Here's how the part is built. I have some questions about the finished solid (model axes, mm). A direction names the side the tool comes from. Give positions to 0.01 mm unless a question says otherwise; leave off trailing zeros. Loops run counter-clockwise (first coordinate to the right, second up) from the corner with the lowest first, then second, coordinate; pieces in that order, holes last. Notation, with made-up numbers: (32.5, -25) - (73.5, -25) arc R15 cw to (73.5, -16) - close; hole circle Ø8 at (24.5, 67.25). An arc over 180 degrees is marked (long way). Return JSON: item names as keys, results as strings. Group by question number.
(1) On a 3-axis mill with a long thin cutter (end or side, diameter ignored), from which of +Z, -Z, +X, -X, +Y, -Y can I reach the whole of each face in a straight line? I mean faces 5 (the flat face through (140, 3.5, -140)), 6 (the conical face through (140.899, 5.791, -140.997)), 7 (the cylindrical face through (1.774, 70.436, -69.048)). Say none if no direction works.
(2) If we section it at A-A (y = 75): Please give me the cut outline in (x, z).
(3) If we section it at C-C (x = 110.5): Please give me the cut outline in (y, z).
(4) If we section it at B-B (z = -75): Please give me the cut outline in (x, y).
(5) If we section it at D-D (x = 25): Please give me the cut outline in (y, z), then the cut area to 3 significant figures.
(6) If we mould it in two halves opening along Z, with no side actions, what happens to faces 1 (the flat face through (74, 3.5, -61)), 2 (the flat face through (74, 77, 0)), 3 (the flat face through (150, 77, -60)), 4 (the cylindrical face through (6.35, 78.77, -143.49))? For each: released by +Z, released by -Z, zero draft, split by the parting line, or undercut.
(7) I need wall thicknesses on probe 1 along X at (y, z) = (120, -70); probe 2 along Z at (x, y) = (89, 30.5); probe 3 along Y at (x, z) = (147.5, -75). Which ranges of each line are inside material? Lowest first, please. Write a range as [from, to].
(8) For P1, Ø1, axis at x = 83.5, z = -70.5, coming from the +Y side; P2, Ø3, axis at x = 149, y = 138, coming from the -Z side; P3, Ø4, axis at y = 1, z = -113.5, coming from the +X side; P4, Ø12, axis at y = 75, z = -75, coming from the +X side, each with a flat end and sliding along its axis, tell me the tip position at first contact or that it passes through.
```python
from build123d import *

# Parameters (mm, degrees)
SKETCH1_W           = 150
SKETCH1_H           = 150
BOSS_EXTRUDE1_DEPTH = 150
SHELL1_T            = -3.5
FILLET2_R           = 10
FILLET3_R           = 10
SKETCH2_R           = 7.5
CUT_EXTRUDE1_DEPTH  = 200
CHAMFER1_SIZE       = 6
CHAMFER2_SIZE       = 6
SKETCH3_W           = 10
SKETCH3_H           = 5
CUT_EXTRUDE2_DEPTH  = 234
SKETCH4_W           = 10
SKETCH4_H           = 5
CUT_EXTRUDE3_DEPTH  = 234
SKETCH5_W           = 40
SKETCH5_H           = 40
CUT_EXTRUDE4_DEPTH  = 10
SKETCH6_W           = 4
SKETCH6_H           = 45
BOSS_EXTRUDE2_DEPTH = 40
FILLET4_R           = 10
SKETCH7_W           = 40
SKETCH7_H           = 40
CUT_EXTRUDE5_DEPTH  = 40


with BuildPart() as part:
    # Sketch1 → Boss-Extrude1 (new body)
    with BuildSketch(Plane(origin=(0, 0, 0), x_dir=(1, 0, 0), z_dir=(0, 1, 0))):
        with Locations((75, 75)):
            Rectangle(SKETCH1_W, SKETCH1_H)
    extrude(amount=BOSS_EXTRUDE1_DEPTH)

    # Shell1
    shell1_openings = [part.faces().sort_by_distance(p)[0] for p in [
        (75, 150, -75),
    ]]
    offset(amount=SHELL1_T, openings=shell1_openings, kind=Kind.INTERSECTION)

    # Fillet2
    fillet2_edges = [part.edges().sort_by_distance(p)[0] for p in [
        (150, 75, -150),
        (150, 75, 0),
        (0, 75, 0),
    ]]
    fillet(fillet2_edges, radius=FILLET2_R)

    # Fillet3
    fillet3_edges = [part.edges().sort_by_distance(p)[0] for p in [
        (3.5, 76.75, -146.5),
        (3.5, 76.75, -3.5),
        (146.5, 76.75, -3.5),
        (146.5, 76.75, -146.5),
        (0, 75, -150),
    ]]
    fillet(fillet3_edges, radius=FILLET3_R)

    # Sketch2 → Cut-Extrude1 (cut)
    with BuildSketch(Plane(origin=(150, 0, 0), x_dir=(0, 0, -1), z_dir=(1, 0, 0))):
        with Locations((75, 75)):
            Circle(SKETCH2_R)
    extrude(amount=-CUT_EXTRUDE1_DEPTH, mode=Mode.SUBTRACT)

    # Chamfer1
    chamfer1_edges = [part.edges().sort_by_distance(p)[0] for p in [
        (75, 0, -150),
        (150, 0, -75),
        (75, 0, 0),
        (2.928932188, 0, -2.928932188),
        (147.071067812, 0, -2.928932188),
        (147.071067812, 0, -147.071067812),
        (0, 0, -75),
        (2.928932188, 0, -147.071067812),
    ]]
    chamfer(chamfer1_edges, length=CHAMFER1_SIZE)

    # Chamfer2
    chamfer2_edges = [part.edges().sort_by_distance(p)[0] for p in [
        (3.5, 3.5, -75),
        (75, 3.5, -3.5),
        (146.5, 3.5, -75),
        (75, 3.5, -146.5),
        (6.428932188, 3.5, -143.571067812),
        (143.571067812, 3.5, -143.571067812),
        (143.571067812, 3.5, -6.428932188),
        (6.428932188, 3.5, -6.428932188),
    ]]
    chamfer(chamfer2_edges, length=CHAMFER2_SIZE)

    # Sketch3 → Cut-Extrude2 (cut)
    with BuildSketch(Plane.ZY):
        with Locations((-128, 138.5)):
            Rectangle(SKETCH3_W, SKETCH3_H)
    extrude(amount=-CUT_EXTRUDE2_DEPTH, mode=Mode.SUBTRACT)

    # Sketch4 → Cut-Extrude3 (cut)
    with BuildSketch(Plane.ZY):
        with Locations((-22, 138.5)):
            Rectangle(SKETCH4_W, SKETCH4_H)
    extrude(amount=-CUT_EXTRUDE3_DEPTH, mode=Mode.SUBTRACT)

    # Sketch5 → Cut-Extrude4 (cut)
    with BuildSketch(Plane(origin=(0, 3.5, 0), x_dir=(1, 0, 0), z_dir=(0, 1, 0))):
        with Locations((120.5, 120.5)):
            Rectangle(SKETCH5_W, SKETCH5_H)
    extrude(amount=-CUT_EXTRUDE4_DEPTH, mode=Mode.SUBTRACT)

    # Sketch6 → Boss-Extrude2 (add)
    with BuildSketch(Plane(origin=(0, 3.5, 0), x_dir=(1, 0, 0), z_dir=(0, 1, 0))):
        with Locations((46.5, 124)):
            Rectangle(SKETCH6_W, SKETCH6_H)
    extrude(amount=BOSS_EXTRUDE2_DEPTH)

    # Fillet4
    # the kernel refuses this fillet: 10 mm, written as the material it adds along each edge
    with BuildSketch(Plane(origin=(48.5, -15.5, -146.5), x_dir=(1, 0, 0), z_dir=(0, 1, 0))) as fillet4_piece_1_section:
        with BuildLine():
            CenterArc((FILLET4_R, -FILLET4_R), FILLET4_R, 90, 90)
            Line((0, -FILLET4_R), (0, 0))
            Line((0, 0), (FILLET4_R, 0))
        make_face()
    fillet4_piece_1 = extrude(amount=59, mode=Mode.PRIVATE)
    fillet4_piece_1 = split(fillet4_piece_1, bisect_by=Plane(origin=(50.679406429, 12.771443898, -156.771443898), z_dir=(0, 0.7071067811865476, 0.7071067811865476)), keep=Keep.TOP, mode=Mode.PRIVATE)
    fillet4_piece_1 = split(fillet4_piece_1, bisect_by=Plane(origin=(50.679406429, 0, -144.176636194), z_dir=(0, 1, 0)), keep=Keep.TOP, mode=Mode.PRIVATE)
    add(fillet4_piece_1)
    with BuildSketch(Plane(origin=(48.5, 3.5, -101.5), x_dir=(1, 0, 0), z_dir=(0, 0, -1))) as fillet4_piece_2_section:
        with BuildLine():
            CenterArc((FILLET4_R, -FILLET4_R), FILLET4_R, 90, 90)
            Line((0, -FILLET4_R), (0, 0))
            Line((0, 0), (FILLET4_R, 0))
        make_face()
    fillet4_piece_2 = extrude(amount=64, mode=Mode.PRIVATE)
    fillet4_piece_2 = split(fillet4_piece_2, bisect_by=Plane(origin=(50.685995649, 5.81247532, -146.5), z_dir=(0, 0, 1)), keep=Keep.TOP, mode=Mode.PRIVATE)
    add(fillet4_piece_2)

    # Sketch7 → Cut-Extrude5 (cut)
    with BuildSketch(Plane(origin=(3.5, 0, 0), x_dir=(0, 0, -1), z_dir=(1, 0, 0))):
        with Locations((116.5, 29.5)):
            Rectangle(SKETCH7_W, SKETCH7_H)
    extrude(amount=-CUT_EXTRUDE5_DEPTH, mode=Mode.SUBTRACT)


solid = part.part
```
Values:
{
 "1": {"face 5": "-Y", "face 6": "+Y", "face 7": "+X, -X"},
 "2": {"outline": "(0, -140) arc R10 ccw to (10, -150) - (140, -150) arc R10 ccw to (150, -140) - (150, -82.5) - (146.5, -82.5) - (146.5, -136.5) arc R10 cw to (136.5, -146.5) - (13.5, -146.5) arc R10 cw to (3.5, -136.5) - (3.5, -82.5) - (0, -82.5) - close; (0, -67.5) - (3.5, -67.5) - (3.5, -13.5) arc R10 cw to (13.5, -3.5) - (136.5, -3.5) arc R10 cw to (146.5, -13.5) - (146.5, -67.5) - (150, -67.5) - (150, -10) arc R10 ccw to (140, 0) - (10, 0) arc R10 ccw to (0, -10) - close"},
 "3": {"outline": "(0, -144) - (6, -150) - (150, -150) - (150, -146.5) - (9.5, -146.5) - (3.5, -140.5) - (0, -140.5) - close; (0, -100.5) - (3.5, -100.5) - (3.5, -9.5) - (9.5, -3.5) - (150, -3.5) - (150, 0) - (6, 0) - (0, -6) - close"},
 "4": {"outline": "(0, 6) - (6, 0) - (144, 0) - (150, 6) - (150, 67.5) - (146.5, 67.5) - (146.5, 9.5) - (140.5, 3.5) - (9.5, 3.5) - (3.5, 9.5) - (3.5, 67.5) - (0, 67.5) - close; (0, 82.5) - (3.5, 82.5) - (3.5, 150) - (0, 150) - close; (146.5, 82.5) - (150, 82.5) - (150, 150) - (146.5, 150) - close"},
 "5": {"outline": "(0, -144) - (6, -150) - (150, -150) - (150, -146.5) - (9.5, -146.5) - (3.5, -140.5) - (3.5, -9.5) - (9.5, -3.5) - (150, -3.5) - (150, 0) - (6, 0) - (0, -6) - close", "area": "1,550 mm2"},
 "6": {"face 1": "undercut", "face 2": "released by +Z", "face 3": "zero draft", "face 4": "undercut"},
 "7": {"probe 1": "[0, 3.5], [146.5, 150]", "probe 2": "[-150, -146.5], [-3.5, 0]", "probe 3": "[3.5, 67.5], [82.5, 150]"},
 "8": {"P1": "y = 3.5", "P2": "z = -146.61", "P3": "x = 147", "P4": "through"}
}
